Design review of the part shown in the three views and the two pictorial views. Dimensions are in mm from the part's minimum x, y and z. A direction names the side the tool comes from. Give positions to 0.01 mm unless a question says otherwise; leave off trailing zeros. Write each loop counter-clockwise with the first axis right and the second up, starting at its lowest first coordinate (ties: lowest second). Pieces come first, ordered by that corner, then holes.
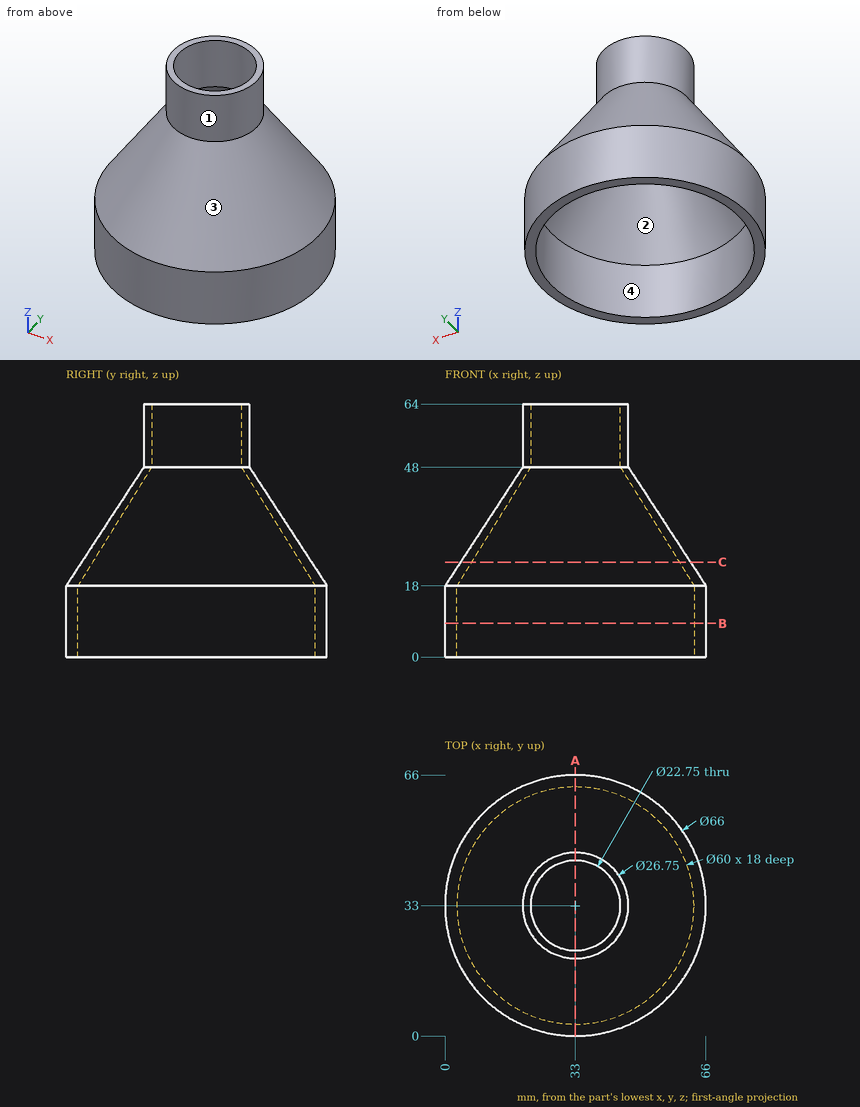
(1) To check wall thickness, follow L1, parallel to Y at x = 33, z = 54.25 (3 decimals); L2, parallel to Y at x = 33, z = 9.25; L3, parallel to Z at x = 56.5, y = 12. State the ranges of each line that lie inside material, in increasing order.
Resolved:
L1: y = 19.625 to 21.625, 44.375 to 46.375
L2: y = 0 to 3, 63 to 66
L3: z = 0 to 20.27
(2) Consider section A-A, the plane x = 33. Give the boundary of the cut face in (y, z) (3 decimals), then the cut area to 3 significant figures.
Resolved:
outline: (0, 0) - (3, 0) - (3, 18) - (21.625, 48) - (21.625, 64) - (19.625, 64) - (19.625, 48) - (0, 18) - close; (44.375, 48) - (63, 18) - (63, 0) - (66, 0) - (66, 18) - (46.375, 48) - (46.375, 64) - (44.375, 64) - close
area: 322 mm2
(3) Consider section B-B, the plane z = 8.5. Give the boundary of the cut face in (x, y).
Resolved:
outline: circle Ø66 at (33, 33); hole circle Ø60 at (33, 33)
(4) Clearance check with flat-ended pins moving along their axes: P1, Ø1, axis at x = 33, y = 10, coming from the -Z side; P2, Ø8, axis at y = 11.5, z = 47.5, coming from the +X side; P3, Ø2, axis at y = 42, z = 47.5, coming from the +X side; P4, Ø1, axis at x = 47.5, y = 12, coming from the +Z side. State where each tip first meets the part, or that it passes through.
Resolved:
P1: stops at z = 28.47
P2: passes through
P3: stops at x = 44.48
P4: stops at z = 30.2
(5) Consider section C-C, the plane z = 24. Give the boundary of the cut face in (x, y) (3 decimals).
Resolved:
outline: circle Ø58.15 at (33, 33); hole circle Ø52.55 at (33, 33)
(6) Tool access review of the marked faces 3 and 4: name each direction out of +Z, -Z, +X, -X, +Y, -Y from which nothing blocks a thin tool from reaching the whole face with its end or side.
Resolved:
face 3: +Z
face 4: -Z
(7) Mouldability with a two-part tool opening along Y and no side actions: class the marked faces 1 and 2 as pulls with the +Y half, pulls with the -Y half, needs draft (parallel to the pull), parting line crosses it, or undercut.
Resolved:
face 1: parting line crosses it
face 2: undercut
